Design review of the part shown in the three views and the two pictorial views. Dimensions are in mm from the part's minimum x, y and z. A direction names the side the tool comes from. Give positions to 0.01 mm unless a question says otherwise; leave off trailing zeros. Order: outer loops, then holes, each group sorted by start corner. A loop starts at its lowest first (then second) coordinate and runs counter-clockwise, first axis right, second up. Notation, with made-up numbers: (48, -10) -> (86, -10) arc R28 ccw to (86, 8) -> close; hole circle Ø3 at (1.5, -13.75). An arc over 180 degrees is marked (long way). Answer in a Markdown table with one row per item. Add a question column.
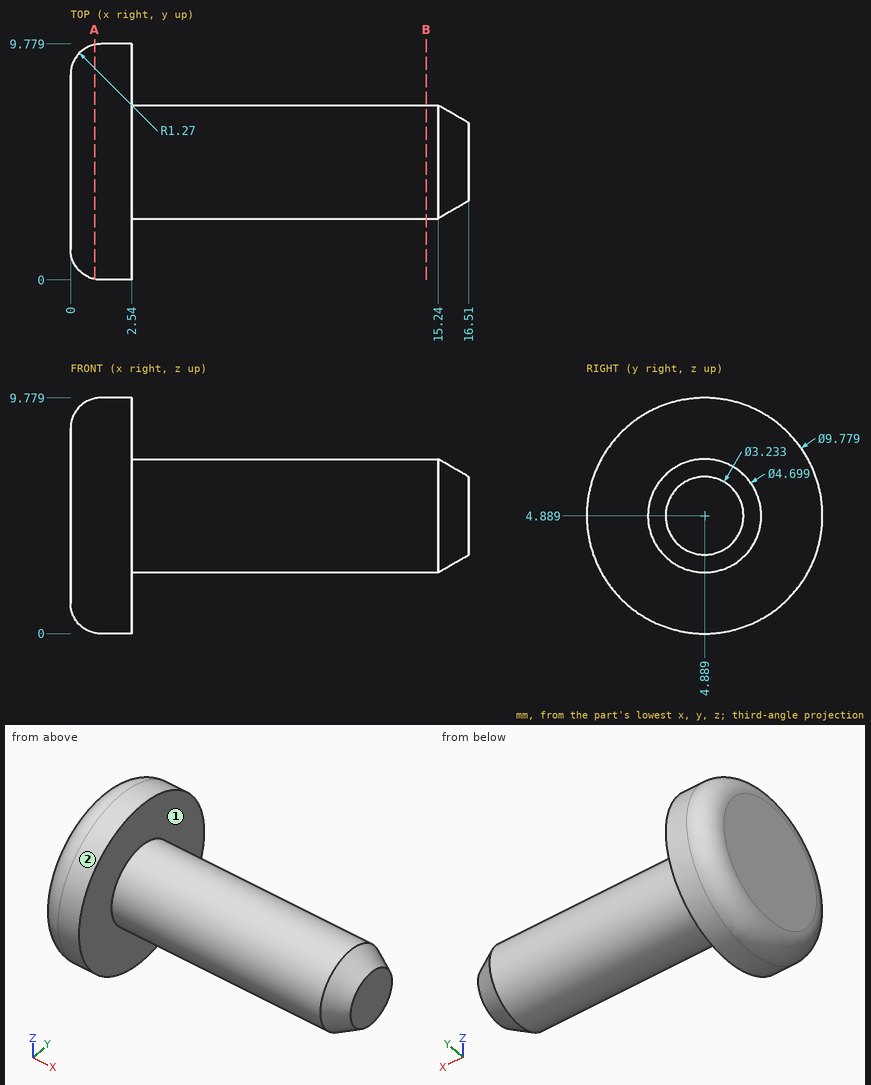
1) Machinability: for the marked faces 1 and 2, which of the approach directions +Z, -Z, +X, -X, +Y, -Y give a long, thin tool a straight path to every point of the face, cutting with its end or side? Answer none if there is none.
2) Add section B-B, the plane x = 14.75. Write out the cut boundary in (y, z).
3) Clearance check with flat-ended pins moving along their axes: P1, Ø3, axis at y = 6.5, z = 3, coming from the +X side; P2, Ø1, axis at x = 8, y = 4, coming from the -Z side; P3, Ø2, axis at x = 1.5, y = 1, coming from the -Z side (1 decimal); P4, Ø5, axis at x = 12, y = 4, coming from the -Z side. State where each tip first meets the part, or that it passes through.
4) Add section A-A, the plane x = 1. Write out the cut boundary in (y, z), and give its area (3 significant figures).
5) For L1, parallel to Z at x = 12.75, y = 5; L2, parallel to X at y = 2, z = 3.25; L3, parallel to Y at x = 7.75, z = 6.75 (1 decimal), list the stretches that pass through material, from the lowest coordinate up.
Verdict:
| question | item | result |
|---|---|---|
| 1 | face 1 | +X |
| 1 | face 2 | +X, -X |
| 2 | outline | circle Ø4.7 at (4.89, 4.89) |
| 3 | P1 | stops at x = 16.51 |
| 3 | P2 | stops at z = 2.57 |
| 3 | P3 | stops at z = 0.9 |
| 3 | P4 | stops at z = 2.54 |
| 4 | outline | circle Ø9.72 at (4.89, 4.89) |
| 4 | area | 74.2 mm2 |
| 5 | L1 | z = 2.54 to 7.24 |
| 5 | L2 | x = 0 to 2.54 |
| 5 | L3 | y = 3.5 to 6.3 |
